Geometry check sheet. Reference: the model listing, model coordinates, mm. A direction names the side the tool comes from. Give positions to 0.01 mm unless a question says otherwise; leave off trailing zeros. Order: outer loops, then holes, each group sorted by start corner. A loop starts at its lowest first (then second) coordinate and runs counter-clockwise, first axis right, second up.
from build123d import *

# Parameters (mm, degrees)
SALIENTE_EXTRUIR1_DEPTH = 9.5
CROQUIS2_R              = 10.875
SALIENTE_EXTRUIR2_DEPTH = 11
CROQUIS3_W              = 26
CROQUIS3_H              = 32
SALIENTE_EXTRUIR3_DEPTH = 3
REDONDEO1_R             = 2.5
CROQUIS4_R              = 11.875
CROQUIS4_R_2            = 9.75
SALIENTE_EXTRUIR4_DEPTH = 1.5
CORTAR_EXTRUIR1_START   = -10
CROQUIS4_3_R            = 9.75
CROQUIS4_3_R_2          = 7.75
CROQUIS4_3_R_3          = 1.375
CORTAR_EXTRUIR1_DEPTH   = 10
CORTAR_EXTRUIR2_REACH   = 33.261
CROQUIS5_R              = 1.15
CHAFL_N1_SIZE           = 1.5
SALIENTE_EXTRUIR5_START = 1
CROQUIS6_R              = 1.375
CROQUIS6_R_2            = 0.5
SALIENTE_EXTRUIR5_DEPTH = 1
CROQUIS6_3_R            = 0.5
SALIENTE_EXTRUIR6_DEPTH = 4
REDONDEO2_R             = 0.25
CROQUIS7_R              = 2.5
CROQUIS7_R_2            = 1.15
SALIENTE_EXTRUIR7_DEPTH = 3


with BuildPart() as part:
    # Croquis1 → Saliente-Extruir1 (new body)
    with BuildSketch(Plane.XY):
        with BuildLine():
            Line((-4.214261501, 6.8), (4.214261501, 6.8))
            ThreePointArc((4.214261501, 6.8), (0, -8), (-4.214261501, 6.8))
        make_face()
    extrude(amount=SALIENTE_EXTRUIR1_DEPTH)

    # Croquis2 → Saliente-Extruir2 (add)
    with BuildSketch(Plane.XY.offset(9.5)):
        Circle(CROQUIS2_R)
    extrude(amount=SALIENTE_EXTRUIR2_DEPTH)

    # Croquis3 → Saliente-Extruir3 (add)
    with BuildSketch(Plane.XY.offset(20.5)):
        Rectangle(CROQUIS3_W, CROQUIS3_H)
    extrude(amount=SALIENTE_EXTRUIR3_DEPTH)

    # Redondeo1
    redondeo1_edges = [part.edges().sort_by_distance(p)[0] for p in [
        (-13, 16, 22),
        (-13, -16, 22),
        (13, -16, 22),
        (13, 16, 22),
    ]]
    fillet(redondeo1_edges, radius=REDONDEO1_R)

    # Croquis4 → Saliente-Extruir4 (add)
    with BuildSketch(Plane.XY.offset(23.5)):
        Circle(CROQUIS4_R)
        Circle(CROQUIS4_R_2, mode=Mode.SUBTRACT)
    extrude(amount=SALIENTE_EXTRUIR4_DEPTH)

    # Croquis4_3 → Cortar-Extruir1 (cut)
    # profile 1 of 4: a face of its own
    with BuildSketch(Plane.XY.offset(23.5).offset(CORTAR_EXTRUIR1_START)):
        Circle(CROQUIS4_3_R)
        Circle(CROQUIS4_3_R_2, mode=Mode.SUBTRACT)
    # profile 2 of 4: a face of its own
    with BuildSketch(Plane.XY.offset(23.5).offset(CORTAR_EXTRUIR1_START)):
        with Locations((4, 0)):
            Circle(CROQUIS4_3_R_3)
    # profile 3 of 4: a face of its own
    with BuildSketch(Plane.XY.offset(23.5).offset(CORTAR_EXTRUIR1_START)):
        with Locations((0, -4)):
            Circle(CROQUIS4_3_R_3)
    # profile 4 of 4: a face of its own
    with BuildSketch(Plane.XY.offset(23.5).offset(CORTAR_EXTRUIR1_START)):
        with Locations((-4, 0)):
            Circle(CROQUIS4_3_R_3)
    extrude(amount=CORTAR_EXTRUIR1_DEPTH, mode=Mode.SUBTRACT)

    # Croquis5 → Cortar-Extruir2 (cut, up to next)
    with BuildSketch(Plane.XY.offset(23.5), mode=Mode.PRIVATE) as cortar_extruir2_sk1:
        with Locations((-9.2, 12.2)):
            Circle(CROQUIS5_R)
    cortar_extruir2_tool1 = extrude(cortar_extruir2_sk1.sketch, amount=-CORTAR_EXTRUIR2_REACH, mode=Mode.PRIVATE) & part.part
    # Croquis5 → Cortar-Extruir2 (cut, up to next)
    with BuildSketch(Plane.XY.offset(23.5), mode=Mode.PRIVATE) as cortar_extruir2_sk2:
        with Locations((9.2, -12.2)):
            Circle(CROQUIS5_R)
    cortar_extruir2_tool2 = extrude(cortar_extruir2_sk2.sketch, amount=-CORTAR_EXTRUIR2_REACH, mode=Mode.PRIVATE) & part.part
    add(cortar_extruir2_tool1.solids().sort_by_distance((-9.2, 12.2, 23.5))[0], mode=Mode.SUBTRACT)
    add(cortar_extruir2_tool2.solids().sort_by_distance((9.2, -12.2, 23.5))[0], mode=Mode.SUBTRACT)

    # Chafl_n1
    chafl_n1_edges = [part.edges().sort_by_distance(p)[0] for p in [
        (-10.35, 12.2, 23.5),
        (8.05, -12.2, 23.5),
    ]]
    chamfer(chafl_n1_edges, length=CHAFL_N1_SIZE)

    # Croquis6 → Saliente-Extruir5 (add)
    # profile 1 of 6: a face of its own
    with BuildSketch(Plane(origin=(0, 0, 0), x_dir=(-1, 0, 0), z_dir=(0, 0, -1)).offset(SALIENTE_EXTRUIR5_START)):
        with Locations(Location((-4, 0, 0), (0, 0, 180))):
            Circle(CROQUIS6_R)
        with Locations((-4, 0)):
            Circle(CROQUIS6_R_2, mode=Mode.SUBTRACT)
    # profile 2 of 6: a face of its own
    with BuildSketch(Plane(origin=(0, 0, 0), x_dir=(-1, 0, 0), z_dir=(0, 0, -1)).offset(SALIENTE_EXTRUIR5_START)):
        with Locations((-4, 0)):
            Circle(CROQUIS6_R_2)
    # profile 3 of 6: a face of its own
    with BuildSketch(Plane(origin=(0, 0, 0), x_dir=(-1, 0, 0), z_dir=(0, 0, -1)).offset(SALIENTE_EXTRUIR5_START)):
        with Locations(Location((4, 0, 0), (0, 0, 180))):
            Circle(CROQUIS6_R)
        with Locations((4, 0)):
            Circle(CROQUIS6_R_2, mode=Mode.SUBTRACT)
    # profile 4 of 6: a face of its own
    with BuildSketch(Plane(origin=(0, 0, 0), x_dir=(-1, 0, 0), z_dir=(0, 0, -1)).offset(SALIENTE_EXTRUIR5_START)):
        with Locations((4, 0)):
            Circle(CROQUIS6_R_2)
    # profile 5 of 6: a face of its own
    with BuildSketch(Plane(origin=(0, 0, 0), x_dir=(-1, 0, 0), z_dir=(0, 0, -1)).offset(SALIENTE_EXTRUIR5_START)):
        with Locations(Location((0, -4, 0), (0, 0, 180))):
            Circle(CROQUIS6_R)
        with Locations((0, -4)):
            Circle(CROQUIS6_R_2, mode=Mode.SUBTRACT)
    # profile 6 of 6: a face of its own
    with BuildSketch(Plane(origin=(0, 0, 0), x_dir=(-1, 0, 0), z_dir=(0, 0, -1)).offset(SALIENTE_EXTRUIR5_START)):
        with Locations((0, -4)):
            Circle(CROQUIS6_R_2)
    extrude(amount=-SALIENTE_EXTRUIR5_DEPTH)

    # Croquis6_3 → Saliente-Extruir6 (add)
    with BuildSketch(Plane(origin=(0, 0, 0), x_dir=(-1, 0, 0), z_dir=(0, 0, -1))):
        with Locations((-4, 0)):
            Circle(CROQUIS6_3_R)
        with Locations((0, -4)):
            Circle(CROQUIS6_3_R)
        with Locations((4, 0)):
            Circle(CROQUIS6_3_R)
    extrude(amount=SALIENTE_EXTRUIR6_DEPTH)

    # Redondeo2
    redondeo2_edges = [part.edges().sort_by_distance(p)[0] for p in [
        (13, 0, 20.5),
        (13, 0, 23.5),
        (-13, 0, 20.5),
        (0, 16, 20.5),
        (0, -16, 20.5),
        (12.267766953, 15.267766953, 20.5),
        (-12.267766953, 15.267766953, 20.5),
        (-12.267766953, -15.267766953, 20.5),
        (12.267766953, -15.267766953, 20.5),
        (0, -16, 23.5),
        (-13, 0, 23.5),
        (0, 16, 23.5),
        (12.267766953, 15.267766953, 23.5),
        (-12.267766953, 15.267766953, 23.5),
        (-12.267766953, -15.267766953, 23.5),
        (12.267766953, -15.267766953, 23.5),
    ]]
    fillet(redondeo2_edges, radius=REDONDEO2_R)

    # Croquis7 → Saliente-Extruir7 (add)
    # profile 1 of 2: a face of its own
    with BuildSketch(Plane(origin=(0, 0, 20.5), x_dir=(-1, 0, 0), z_dir=(0, 0, -1))):
        with Locations(Location((-9.2, -12.2, 0), (0, 0, 180))):
            Circle(CROQUIS7_R)
        with Locations(Location((-9.2, -12.2, 0), (0, 0, 180))):
            Circle(CROQUIS7_R_2, mode=Mode.SUBTRACT)
    # profile 2 of 2: a face of its own
    with BuildSketch(Plane(origin=(0, 0, 20.5), x_dir=(-1, 0, 0), z_dir=(0, 0, -1))):
        with Locations(Location((9.2, 12.2, 0), (0, 0, 180))):
            Circle(CROQUIS7_R)
        with Locations(Location((9.2, 12.2, 0), (0, 0, 180))):
            Circle(CROQUIS7_R_2, mode=Mode.SUBTRACT)
    extrude(amount=SALIENTE_EXTRUIR7_DEPTH)


solid = part.part
Item 1: Sectioned sample at C-C (z = -0.5). Enter the section's corners in (x, y) (3 decimals).
Reported:
outline: circle Ø2.75 at (-4, 0); circle Ø2.75 at (0, -4); circle Ø2.75 at (4, 0)
Item 2: Sectioned sample at A-A (z = 16). Enter the section's corners in (x, y) (3 decimals).
Reported:
outline: circle Ø21.75 at (0, 0); circle Ø15.5 at (0, 0); hole circle Ø19.5 at (0, 0); hole circle Ø2.75 at (-4, 0); hole circle Ø2.75 at (0, -4); hole circle Ø2.75 at (4, 0)
Item 3: Set-up check for faces 5 (the flat face through (10, -11, 17.5)), 6 (the flat face through (2, 12, 23.5)), 7 (the flat face through (-8, 13, 17.5)), 8 (the cylindrical face through (0, -8, 5)): record each of +Z, -Z, +X, -X, +Y, -Y from which the full face is reachable in a straight line by a thin tool's end or side.
Reported:
face 5: -Z, +X, -Y
face 6: +Z
face 7: -Z, -X, +Y
face 8: -Z
Item 4: Gauge pin test, flat ends, axial feed: pin 1 (4 mm diameter, centred on y = 12, z = 13.5, fed in from +X); pin 2 (2 mm diameter, centred on x = -4.5, y = 0, fed in from +Z); pin 3 (5 mm diameter, centred on y = 11, z = 16, fed in from +X). Record the tip position at first contact, or that the pin passes through.
Reported:
pin 1: stops at x = 4.27
pin 2: stops at z = 23.5
pin 3: stops at x = 6.78
Item 5: Draft check along X on faces 1 (the cylindrical face through (12.248, -15.287, 22.018)), 2 (the flat face through (0, -4, 13.5)), 3 (the flat face through (0, 6.8, 5)), 4 (the flat face through (4, 1, -1)). Enter one of: released by +X, released by -X, zero draft, split by the parting line, or undercut.
Reported:
face 1: released by +X
face 2: undercut
face 3: zero draft
face 4: undercut
Item 6: Sectioned sample at D-D (z = 12.75). Enter the section's corners in (x, y) (3 decimals), and give its area (3 significant figures).
Reported:
outline: circle Ø21.75 at (0, 0)
area: 372 mm2
Item 7: Scan lines: L1, parallel to Y at x = 0, z = 18.75 (3 decimals); L2, parallel to X at y = -12.2, z = 20.7; L3, parallel to X at y = -12.2, z = 20.45. Record each from-to range of solid material in increasing order.
Reported:
L1: y = -10.875 to -9.75, -7.75 to -5.375, -2.625 to 7.75, 9.75 to 10.875
L2: x = -12.99 to 8.05, 10.35 to 12.99
L3: x = 6.7 to 8.05, 10.35 to 11.7
